```python
from build123d import *

# Parameters (mm, degrees)
EXTRUDE_4_DEPTH     = 3
EXTRUDE_6_DEPTH     = 43
EXTRUDE_7_DEPTH     = 40
EXTRUDE_8_DEPTH     = 40
SKETCH_14_R         = 1.25
CUT_EXTRUDE_3_DEPTH = 10


with BuildPart() as part:
    # 草图1 → 凸台-拉伸4 (new body)
    with BuildSketch(Plane.XY):
        with BuildLine():
            ThreePointArc((11.999755772, 64.190702015), (7.19287537, 69.699227744), (0.441332655, 66.894477154))
            Line((0.441332655, 66.894477154), (-16.87917542, 36.894477154))
            Line((-16.87917542, 36.894477154), (-16.87917542, -3.105522846))
            Line((-16.87917542, -3.105522846), (-5.332170037, -23.105522846))
            Line((-5.332170037, -23.105522846), (9.992741519, -33.105522846))
            Line((9.992741519, -33.105522846), (11.999755772, -30.029791253))
            Line((11.999755772, -30.029791253), (-6.87917542, -3.105522846))
            Line((-6.87917542, -3.105522846), (-6.87917542, 14.190702015))
            Line((-6.87917542, 14.190702015), (-6.87917542, 24.190702015))
            Line((-6.87917542, 24.190702015), (10.114332844, 34.190702015))
            Line((10.114332844, 34.190702015), (11.999755772, 64.190702015))
        make_face()
    extrude(amount=EXTRUDE_4_DEPTH)

    # 草图6 → 凸台-拉伸6 (add)
    with BuildSketch(Plane(origin=(0, 0, 0), x_dir=(-1, 0, 0), z_dir=(0, 0, -1))):
        Polygon((6.87917542, 24.190702015), (8.248400541, 24.190702015), (8.248400541, -3.145484966), (-10.996248645, -31.567657049), (-11.999755772, -30.029791253), (6.87917542, -3.105522846), align=None)
    extrude(amount=-EXTRUDE_6_DEPTH)

    # 草图9 → 凸台-拉伸7 (add)
    with BuildSketch(Plane.XY.offset(3)):
        Polygon((-8.248400541, 24.190702015), (-6.858844556, 26.362086453), (8.966526684, 35.828548473), (10.114332844, 34.190702015), (-6.87917542, 24.190702015), align=None)
    extrude(amount=EXTRUDE_7_DEPTH)

    # 草图11 → 凸台-拉伸8 (add)
    with BuildSketch(Plane.XY.offset(3)):
        Polygon((8.966526684, 35.828548473), (10.756094136, 64.281113509), (11.999755772, 64.190702015), (10.114332844, 34.190702015), align=None)
    extrude(amount=EXTRUDE_8_DEPTH)

    # 草图14 → 切除-拉伸3 (cut)
    with BuildSketch(Plane(origin=(0, 0, 0), x_dir=(-1, 0, 0), z_dir=(0, 0, -1))):
        with Locations((-2.591697764, 54.404600603)):
            Circle(SKETCH_14_R)
        with Locations((-5.784422652, 63.881230161)):
            Circle(SKETCH_14_R)
    extrude(amount=-CUT_EXTRUDE_3_DEPTH, mode=Mode.SUBTRACT)


solid = part.part
```
Part model, mm, in its own coordinate system. A direction names the side the tool comes from. Round coordinates to 2 decimals unless told otherwise and drop trailing zeros. Order: outer loops, then holes, each group sorted by start corner. A loop starts at its lowest first (then second) coordinate and runs counter-clockwise, first axis right, second up. Notation, with made-up numbers: M -26.5,43.5 L 24.5,43.5 A19 ccw 24.5,70.5 Z; hole C 38,82 d4. An arc over 180 degrees is marked long. Answer in a Markdown table with one row per item. Add a question column.
Q1. Cut at A-A on x = 5.5. Give the cut face in (y, z), and give its area (3 significant figures).
Q2. Cut at B-B on z = 24.5. Give the cut face in (x, y), and give its area (3 significant figures).
Q3. Wall check: L1, parallel to Z at x = -1.25, y = 54.5; L2, parallel to Y at x = -3, z = 39.5; L3, parallel to X at y = 23.5, z = 15. Give the ranges that are in metal, low to high. Write a range as from..to.
Q4. 3-axis set-ups, long thin cutter, end or side, ignore diameter. For faces 4 (the face through (1.24, -17.16, 22.72)), 5 (the face through (2.692, -16.756, 21.199)), 6 (the face through (9.85, 49.86, 22.72)): which of +Z, -Z, +X, -X, +Y, -Y reach the whole face in a straight line?
Q5. Cut at C-C on x = -4.25. Give the cut face in (y, z).
Q6. Pin check, flat tips, straight feed: pin 1 (2 mm diameter, centred on x = 1, z = 11, fed in from -Y); pin 2 (13.5 mm diameter, centred on y = 4.5, z = 28, fed in from -X); pin 3 (1 mm diameter, centred on x = 7.5, z = 8, fed in from +Y). Stop position of each tip, or through.
Q7. Cut at D-D on y = 3.5. Give the cut face in (x, z).
Q8. Mould opens along Y. For faces 1 (the face through (-6, 31, 3)), 2 (the face through (-7.563, 25.261, 22.72)), 3 (the face through (1.737, 29.261, 21.199)) say: +Y half, -Y half, draft (parallel to the pull), parting line (faces both ways), or undercut.
Established:
| question | item | result |
|---|---|---|
| 1 | outline | M -30.17,0 L -20.76,0 L -20.76,43 L -23.45,43 L -23.45,3 L -30.17,3 Z; M 31.48,0 L 62.66,0 L 62.66,3 L 33.75,3 L 33.75,43 L 31.48,43 Z; M 65.1,0 L 69.86,0 L 69.86,3 L 65.1,3 Z |
| 1 | area | 335 mm2 |
| 2 | outline | M -8.25,-3.15 L 11,-31.57 L 12,-30.03 L -6.88,-3.11 L -6.88,24.19 L 10.11,34.19 L 12,64.19 L 10.76,64.28 L 8.97,35.83 L -6.86,26.36 L -8.25,24.19 Z |
| 2 | area | 160 mm2 |
| 3 | L1 | z = 0..3 |
| 3 | L2 | y = -10.9..-8.64, 26.47..28.67 |
| 3 | L3 | x = -8.25..-6.88 |
| 4 | face 4 | +Z, -X, -Y |
| 4 | face 5 | +Z, -Z, +X |
| 4 | face 6 | +Z, -X, +Y |
| 5 | outline | M -23.81,0 L -6.86,0 L -6.86,43 L -9.05,43 L -9.05,3 L -23.81,3 Z; M 25.74,0 L 58.77,0 L 58.77,3 L 27.92,3 L 27.92,43 L 25.74,43 Z |
| 6 | pin 1 | stops at y = -18.28 |
| 6 | pin 2 | stops at x = -8.25 |
| 6 | pin 3 | stops at y = 35.25 |
| 7 | outline | M -16.88,0 L -6.88,0 L -6.88,43 L -8.25,43 L -8.25,3 L -16.88,3 Z |
| 8 | face 1 | draft |
| 8 | face 2 | +Y half |
| 8 | face 3 | undercut |
